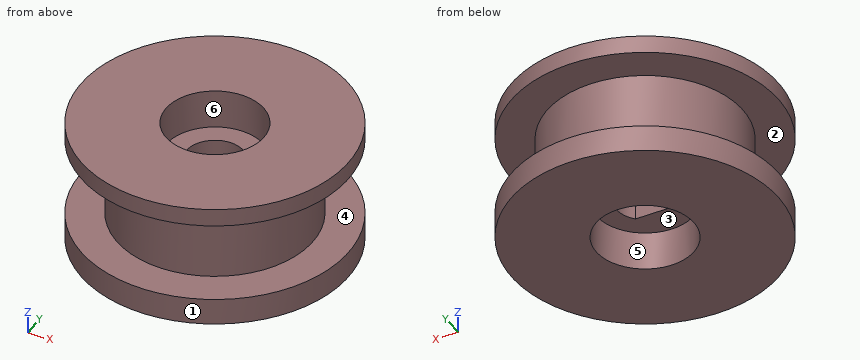
from build123d import *

# Parameters (mm, degrees)
SKETCH2_R           = 3
CUT_EXTRUDE1_DEPTH  = 2
SKETCH3_R           = 2.25
SKETCH3_R_2         = 1.25
BOSS_EXTRUDE1_DEPTH = 5
SKETCH4_R           = 1.6
CUT_EXTRUDE2_DEPTH  = 10
BOSS_EXTRUDE2_DEPTH = 7
SKETCH6_R           = 2.75
CUT_EXTRUDE4_DEPTH  = 2.2
CUT_EXTRUDE5_START  = -2.2
SKETCH7_R           = 2.75
CUT_EXTRUDE5_DEPTH  = 2.2


with BuildPart() as part:
    # Sketch1 → Revolve1 (revolve)
    with BuildSketch(Plane(origin=(0, 0, 0), x_dir=(1, 0, 0), z_dir=(0, 1, 0))):
        Polygon((1.25, 0), (7.5, 0), (7.5, 1), (5.5, 1), (5.5, 5.5), (7.5, 5.5), (7.5, 7), (3, 7), (3, 9), (2.25, 9), (2.25, 2), (1.25, 2), align=None)
    revolve(axis=Axis((0, 0, 0), (0, 0, -1)))

    # Sketch2 → Cut-Extrude1 (cut)
    with BuildSketch(Plane(origin=(0, 0, -9), x_dir=(-1, 0, 0), z_dir=(0, 0, -1))):
        Circle(SKETCH2_R)
    extrude(amount=-CUT_EXTRUDE1_DEPTH, mode=Mode.SUBTRACT)

    # Sketch3 → Boss-Extrude1 (add)
    with BuildSketch(Plane(origin=(0, 0, -2), x_dir=(-1, 0, 0), z_dir=(0, 0, -1))):
        Circle(SKETCH3_R)
        with Locations(Location((0, 0, 0), (0, 0, 180))):
            Circle(SKETCH3_R_2, mode=Mode.SUBTRACT)
    extrude(amount=BOSS_EXTRUDE1_DEPTH)

    # Sketch4 → Cut-Extrude2 (cut)
    with BuildSketch(Plane(origin=(0, 0, -7), x_dir=(-1, 0, 0), z_dir=(0, 0, -1))):
        Circle(SKETCH4_R)
    extrude(amount=-CUT_EXTRUDE2_DEPTH, mode=Mode.SUBTRACT)

    # Sketch5 → Boss-Extrude2 (add)
    with BuildSketch(Plane(origin=(0, 0, -7), x_dir=(-1, 0, 0), z_dir=(0, 0, -1))):
        with BuildLine():
            Line((-1.161895004, -1.1), (1.161895004, -1.1))
            ThreePointArc((1.161895004, -1.1), (0, -1.6), (-1.161895004, -1.1))
        make_face()
    extrude(amount=-BOSS_EXTRUDE2_DEPTH)

    # Sketch6 → Cut-Extrude4 (cut)
    with BuildSketch(Plane.XY):
        Circle(SKETCH6_R)
    extrude(amount=-CUT_EXTRUDE4_DEPTH, mode=Mode.SUBTRACT)

    # Sketch7 → Cut-Extrude5 (cut)
    with BuildSketch(Plane(origin=(0, 0, -7), x_dir=(-1, 0, 0), z_dir=(0, 0, -1)).offset(CUT_EXTRUDE5_START)):
        with Locations(Location((0, 0, 0), (0, 0, 180))):
            Circle(SKETCH7_R)
    extrude(amount=CUT_EXTRUDE5_DEPTH, mode=Mode.SUBTRACT)


solid = part.part
Here's how the part is built. I have some questions about the finished solid (model axes, mm). Face numbers are marked on the shaded views. A direction names the side the tool comes from. Round coordinates to 2 decimals unless told otherwise and drop trailing zeros. Loops run counter-clockwise (first coordinate to the right, second up) from the corner with the lowest first, then second, coordinate; pieces in that order, holes last. Notation, with made-up numbers: (79, -16) - (90, -16) arc R20 ccw to (90, 13) - close; hole circle Ø5 at (13, 69.5). An arc over 180 degrees is marked (long way). One line per question, with ' | ' between items. Start each with the question number.
Q1. I want a section at A-A (x = 0). Write out the boundary of the cut face in (y, z).
Q2. We'd pull the mould along Z, two halves only. Please class the marked faces 1, 2 and 3: +Z half, -Z half, draft (parallel to the pull), parting line (faces both ways), or undercut.
Q3. Will these pins go through, and if not, where does the flat tip stop? pin 1 (3 mm diameter, centred on y = -1, z = -3.5, fed in from -X); pin 2 (3 mm diameter, centred on x = 0, y = 0, fed in from +Z); pin 3 (0.7 mm diameter, centred on x = 0, z = -3, fed in from +Y).
Q4. I want a section at B-B (y = 0). Write out the boundary of the cut face in (x, z).
Q5. Please list where these lines run through material, in increasing order: line 1 (Y direction, x = 0, z = -0.55); line 2 (Z direction, x = -3.5, y = -5.5); line 3 (Y direction, x = 0, z = -1.45). Write a range as [from, to].
Q6. I want a section at C-C (z = -3). Write out the boundary of the cut face in (x, y), then the cut area to 3 significant figures.
Q7. For the marked faces 4, 5 and 6, which set-ups out of +Z, -Z, +X, -X, +Y, -Y let a thin tool reach every point of the face, with its end or its side?
Q8. I want a section at D-D (x = -5.25). Write out the boundary of the cut face in (y, z), then the cut area to 3 significant figures.
Response values:
1) outline: (-7.5, -7) - (-2.75, -7) - (-2.75, -4.8) - (-1.1, -4.8) - (-1.1, -2.2) - (-2.75, -2.2) - (-2.75, 0) - (-7.5, 0) - (-7.5, -1) - (-5.5, -1) - (-5.5, -5.5) - (-7.5, -5.5) - close; (1.6, -4.8) - (2.75, -4.8) - (2.75, -7) - (7.5, -7) - (7.5, -5.5) - (5.5, -5.5) - (5.5, -1) - (7.5, -1) - (7.5, 0) - (2.75, 0) - (2.75, -2.2) - (1.6, -2.2) - close
2) face 1: draft | face 2: undercut | face 3: -Z half
3) pin 1: stops at x = -5.5 | pin 2: stops at z = -2.2 | pin 3: stops at y = 5.5
4) outline: (-7.5, -7) - (-2.75, -7) - (-2.75, -4.8) - (-1.6, -4.8) - (-1.6, -2.2) - (-2.75, -2.2) - (-2.75, 0) - (-7.5, 0) - (-7.5, -1) - (-5.5, -1) - (-5.5, -5.5) - (-7.5, -5.5) - close; (1.6, -4.8) - (2.75, -4.8) - (2.75, -7) - (7.5, -7) - (7.5, -5.5) - (5.5, -5.5) - (5.5, -1) - (7.5, -1) - (7.5, 0) - (2.75, 0) - (2.75, -2.2) - (1.6, -2.2) - close
5) line 1: y = [-7.5, -2.75], [2.75, 7.5] | line 2: z = [-7, -5.5], [-1, 0] | line 3: y = [-5.5, -2.75], [2.75, 5.5]
6) outline: circle Ø11 at (0, 0); hole (-1.16, -1.1) - (1.16, -1.1) arc R1.6 ccw (long way) to start | area: 87.8 mm²
7) face 4: none | face 5: -Z | face 6: +Z
8) outline: (-5.36, -7) - (5.36, -7) - (5.36, -5.5) - (1.64, -5.5) - (1.64, -1) - (5.36, -1) - (5.36, 0) - (-5.36, 0) - (-5.36, -1) - (-1.64, -1) - (-1.64, -5.5) - (-5.36, -5.5) - close | area: 41.5 mm²
